from build123d import *

# Parameters (mm, degrees)
ESQUISSE1_W             = 45
ESQUISSE1_H             = 20
BOSS_EXTRU_1_DEPTH      = 3
ESQUISSE2_W             = 15
ESQUISSE2_H             = 20
BOSS_EXTRU_2_DEPTH      = 5
ESQUISSE3_W             = 45
ESQUISSE3_H             = 15
BOSS_EXTRU_3_DEPTH      = 2
ENL_V_MAT_EXTRU_1_REACH = 46.348
ESQUISSE4_R             = 3
BOSS_EXTRU_4_DEPTH      = 5


with BuildPart() as part:
    # Esquisse1 → Boss.-Extru.1 (new body)
    with BuildSketch(Plane.XY):
        with Locations((1.348933413, 4.924242424)):
            Rectangle(ESQUISSE1_W, ESQUISSE1_H)
    extrude(amount=BOSS_EXTRU_1_DEPTH)

    # Esquisse2 → Boss.-Extru.2 (add)
    with BuildSketch(Plane.ZY.offset(21.151066587)):
        with Locations((-4.5, 4.924242424)):
            Rectangle(ESQUISSE2_W, ESQUISSE2_H)
    extrude(amount=-BOSS_EXTRU_2_DEPTH)

    # Esquisse3 → Boss.-Extru.3 (add)
    with BuildSketch(Plane.XZ.offset(5.075757576)):
        with Locations((1.348933413, -4.5)):
            Rectangle(ESQUISSE3_W, ESQUISSE3_H)
    extrude(amount=BOSS_EXTRU_3_DEPTH)

    # Esquisse4 → Enlèv. mat.-Extru.1 (cut, up to next)
    with BuildSketch(Plane(origin=(-16.151066587, 0, 0), x_dir=(0, 0, -1), z_dir=(1, 0, 0)), mode=Mode.PRIVATE) as enl_v_mat_extru_1_sk1:
        with Locations(Location((6.311557668, 5.877767498, 0), (0, 0, 90))):
            Circle(ESQUISSE4_R)
    enl_v_mat_extru_1_tool1 = extrude(enl_v_mat_extru_1_sk1.sketch, amount=-ENL_V_MAT_EXTRU_1_REACH, mode=Mode.PRIVATE) & part.part
    add(enl_v_mat_extru_1_tool1.solids().sort_by_distance((-16.151067, 5.877767, -6.311558))[0], mode=Mode.SUBTRACT)

    # Esquisse5 → Boss.-Extru.4 (add)
    with BuildSketch(Plane(origin=(-16.151066587, 0, 0), x_dir=(0, 0, -1), z_dir=(1, 0, 0))):
        Polygon((6.61719562, 9.041849495), (5.191621887, 2.399624229), (5.877852712, 2.252343371), (7.335036292, 9.041849495), align=None)
    extrude(amount=-BOSS_EXTRU_4_DEPTH)


solid = part.part
Check sheet for the modelled part. Datum: model origin and axes. Units: mm. A direction names the side the tool comes from. Give positions to 0.01 mm unless a question says otherwise; leave off trailing zeros. Write each loop counter-clockwise with the first axis right and the second up, starting at its lowest first coordinate (ties: lowest second). Pieces come first, ordered by that corner, then holes. Notation, with made-up numbers: (-38.5, -7) -> (-30.5, -7) arc R12 cw to (-30.5, 15) -> close; hole circle Ø5 at (54.25, 49). An arc over 180 degrees is marked (long way). Use one line per item in the form item = value. Start each with the question number.
1. Access from +Z, -Z, +X, -X, +Y, -Y to the whole of each face (thin tool, end or side, straight path). Record for faces 5 (the flat face through (-18.616, 5.995, -5.963)), 6 (the flat face through (1, -7.076, -4)), 7 (the flat face through (-16.151, 5, -6)).
2. Section check A-A (y = 12). Record the cut outline in (x, z).
3. Go/stop test with flat-tipped pins: P1, Ø3.5, axis at x = 7, z = -4, coming from the +Y side; P2, Ø2, axis at x = 11, y = 10, coming from the -Z side. Record where each tip stops, or that it passes through.
4. Section check B-B (z = -1). Record the cut outline in (x, y).
5. Section check C-C (z = -4.75). Record the cut outline in (x, y), and give its area (3 significant figures).
6. Thickness scan on line 1 along Z through (x, y) = (10, 11.5); line 2 along Y through (x, z) = (20, -5); line 3 along X through (y, z) = (2.75, -3.75). Record the ranges inside material, lowest first. Write a range as from..to.
7. Mould release check, pull along Z, two halves, no side actions. Record for faces 1 (the cylindrical face through (-18.6, 6.6, -3.4)), 2 (the flat face through (1, 4, 3)), 3 (the cylindrical face through (-18.62, 5.19, -9.23)), 4 (the flat face through (4, 5, 0)): pulls with the +Z half, pulls with the -Z half, needs draft (parallel to the pull), parting line crosses it, or undercut.
Conclusion:
q1.face_5 = +X, -X
q1.face_6 = +Z, -Z, +X, -X, -Y
q1.face_7 = -Z, +X, +Y
q2.outline = (-21.15, -12) -> (-16.15, -12) -> (-16.15, 0) -> (23.85, 0) -> (23.85, 3) -> (-21.15, 3) -> close
q3.P1 = -5.08
q3.P2 = 0
q4.outline = (-21.15, -7.08) -> (23.85, -7.08) -> (23.85, -5.08) -> (-16.15, -5.08) -> (-16.15, 14.92) -> (-21.15, 14.92) -> close
q5.outline = (-21.15, -7.08) -> (23.85, -7.08) -> (23.85, -5.08) -> (-16.15, -5.08) -> (-16.15, 3.32) -> (-21.15, 3.32) -> close; (-21.15, 8.44) -> (-16.15, 8.44) -> (-16.15, 14.92) -> (-21.15, 14.92) -> close
q5.area = 164 mm²
q6.line_1 = 0..3
q6.line_2 = -7.08..-5.08
q6.line_3 = -21.15..-16.15
q7.face_1 = undercut
q7.face_2 = pulls with the +Z half
q7.face_3 = undercut
q7.face_4 = pulls with the -Z half
